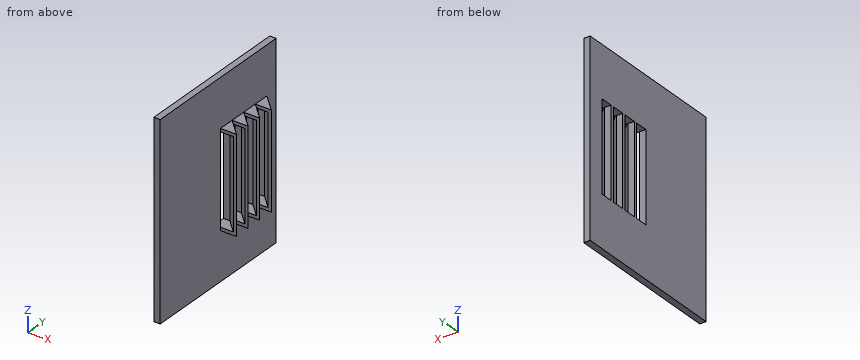
Autodesk Inventor part; units mm, degrees
ref_plane "Work Plane5" through (0, 0, 0) normal (0, 0, 1) x (1, 0, 0)
ref_plane "YZ Plane" through (0, 0, 0) normal (1, 0, 0) x (0, 1, 0)
ref_plane "XZ Plane" through (0, 0, 0) normal (0, 1, 0) x (-1, 0, 0)
sketch "Sketch1" plane through (0, 0, 0) normal (1, 0, 0) x (0, 1, 0)
  line L0 (0, 76.2) -> (127, 76.2)
  line L1 (127, 76.2) -> (127, -76.2)
  line L2 (127, -76.2) -> (0, -76.2)
  line L3 (0, -76.2) -> (0, 76.2)
  point P0 (0, 0)
  point P1 (0, 0)
  dimension "d0" = 127
  dimension "d1" = 152.4
extrude "Extrusion1" add sketch "Sketch1" along normal blind 5.08
sketch "Sketch11" plane through (0, 0, 0) normal (0, 0, 1) x (1, 0, 0)
  line L0 (5.08, 127) -> (5.08, 0)
  line L1 (5.08, 0) -> (5.08, 127)
  line L2 (5.08, 116.84) -> (5.08, 104.14)
  line L3 (5.08, 104.14) -> (17.78, 104.14)
  line L4 (17.78, 104.14) -> (5.08, 116.84)
  line L5 (0, 127) -> (5.08, 127)
  point P0 (0, 0)
  point P1 (2.54, 127)
  dimension "d31" = 10.16
  dimension "d32" = 12.7
  dimension "d33" = 45
extrude "Extrusion5" add sketch "Sketch11" along normal mid plane 76.2
ref_plane "Work Plane5" through (0, 0, 0) normal (0, 0, 1) x (1, 0, 0)
sketch "Sketch17" plane through (0, 0, 0) normal (0, 0, 1) x (1, 0, 0)
  line L0 (0, 0) -> (0, 127)
  line L1 (17.78, 104.14) -> (5.08, 104.14)
  line L2 (15.24, 104.14) -> (0, 104.14)
  line L3 (0, 114.3) -> (5.08, 114.3)
  line L4 (5.08, 0) -> (5.08, 127)
  line L5 (5.08, 114.3) -> (15.24, 104.14)
  line L6 (0, 104.14) -> (0, 114.3)
  dimension "d45" = 10.16
  dimension "d46" = 45
extrude "Extrusion6" cut sketch "Sketch17" along normal mid plane 71.12
pattern_linear "Rectangular Pattern4" count 4 spacing 12.7 along (0, -1, 0) of "Extrusion5", "Extrusion6"
Read the model definition and answer for the solid it produces. Units are mm, in the model's axes. Round coordinates to 2 decimals unless told otherwise and drop trailing zeros. Write each loop counter-clockwise with the first axis right and the second up, starting at its lowest first coordinate (ties: lowest second). Pieces come first, ordered by that corner, then holes.
1. Given pin 1 Ø2 at (y, z) = (98.5, -29) entering from +X; pin 2 Ø8 at (x, y) = (12.5, 103.5) entering from +Z; pin 3 Ø4 at (x, z) = (10, 17.5) entering from -Y, each flat-ended and moving along its own axis, determine where each tip first touches the part or whether it passes through.
2. The part is cut by section C-C, the plane x = 2.5. Determine the outline of the cut face in (y, z), then the cut area to 3 significant figures.
3. The part is cut by section D-D, the plane y = 70.5. Determine the outline of the cut face in (x, z).
4. Straight lines are drawn through the part: L1, parallel to Y at x = 3.5, z = 26.5; L2, parallel to Z at x = 2.75, y = 67; L3, parallel to Y at x = 5.25, z = 16. For each, find the intervals that lie inside material, in ascending order.
5. The part is cut by section A-A, the plane x = 10.75. State how many separate pieces and enclosed holes the cut face has, then the cut area to 3 significant figures.
Values:
1. pin 1: stops at x = 11.72
1. pin 2: stops at z = 38.1
1. pin 3: stops at y = 69.28
2. outline: (0, -76.2) - (127, -76.2) - (127, 76.2) - (0, 76.2) - close; hole (66.04, -35.56) - (76.2, -35.56) - (76.2, 35.56) - (66.04, 35.56) - close; hole (78.74, -35.56) - (88.9, -35.56) - (88.9, 35.56) - (78.74, 35.56) - close; hole (91.44, -35.56) - (101.6, -35.56) - (101.6, 35.56) - (91.44, 35.56) - close; hole (104.14, -35.56) - (114.3, -35.56) - (114.3, 35.56) - (104.14, 35.56) - close
2. area: 16,500 mm2
3. outline: (0, -76.2) - (5.08, -76.2) - (5.08, -38.1) - (13.32, -38.1) - (13.32, 38.1) - (5.08, 38.1) - (5.08, 76.2) - (0, 76.2) - (0, 35.56) - (10.78, 35.56) - (10.78, -35.56) - (0, -35.56) - close
4. L1: y = 0 to 66.04, 76.2 to 78.74, 88.9 to 91.44, 101.6 to 104.14, 114.3 to 127
4. L2: z = -76.2 to -35.56, 35.56 to 76.2
4. L3: y = 76.03 to 78.57, 88.73 to 91.27, 101.43 to 103.97, 114.13 to 116.67
5. separate pieces: 4
5. enclosed holes: 0
5. area: 865 mm2
